```python
from build123d import *

# Parameters (mm, degrees)
SKETCH_1_R      = 98
SKETCH_1_R_2    = 47
EXTRUDE_1_DEPTH = 20
SKETCH_2_W      = 142.329371157
SKETCH_2_H      = 73.846071027
EXTRUDE_2_DEPTH = 15
FILLET_1_R      = 22


with BuildPart() as part:
    # 草图1 → 凸台-拉伸1 (new body)
    with BuildSketch(Plane.XY):
        with Locations((-11.887359686, -2.794806673)):
            Circle(SKETCH_1_R)
        with Locations((-11.887359686, -2.794806673)):
            Circle(SKETCH_1_R_2, mode=Mode.SUBTRACT)
    extrude(amount=EXTRUDE_1_DEPTH)

    # 草图2 → 凸台-拉伸2 (add)
    with BuildSketch(Plane.XY.offset(20)):
        with Locations((-173.83028852, -2.794806673)):
            Rectangle(SKETCH_2_W, SKETCH_2_H)
    extrude(amount=-EXTRUDE_2_DEPTH)

    # 圆角1
    fillet_1_edges = [part.edges().sort_by_distance(p)[0] for p in [
        (-102.665602941, 34.128228841, 12.5),
        (-102.665602941, -39.717842186, 12.5),
    ]]
    fillet(fillet_1_edges, radius=FILLET_1_R)


solid = part.part
```
Read the model definition and answer for the solid it produces. Units are mm, in the model's axes. A direction names the side the tool comes from. Give positions to 0.01 mm unless a question says otherwise; leave off trailing zeros. Loops run counter-clockwise (first coordinate to the right, second up) from the corner with the lowest first, then second, coordinate; pieces in that order, holes last.
Item 1: For faces 4 (the flat face through (-182, -39.718, 13)), 5 (the flat face through (-244.995, -3, 13)), 6 (the flat face through (-182, 34.128, 13)), determine the directions among +Z, -Z, +X, -X, +Y, -Y from which every point of the face is accessible in a straight line to the end or side of a thin tool.
Item 2: Each of these flat-tipped pins is pushed along its axis until it touches: pin 1 Ø3 at (y, z) = (69.5, 3) entering from -X; pin 2 Ø8 at (x, y) = (-198, 14.5) entering from -Z; pin 3 Ø3 at (x, z) = (-168.5, 4.5) entering from +Y. Where does it stop, or does it pass through?
Item 3: Find the intervals of material crossed by line 1 along Y through (x, z) = (-54, 8); line 2 along X through (y, z) = (-25.5, 1.75); line 3 along Y through (x, z) = (-0.5, 15.75), in increasing order.
Item 4: The part is cut by section A-A (x = 24). Write down the section's boundary in (y, z), and give its area (3 significant figures).
Item 5: The part is cut by section D-D (x = -199). Write down the section's boundary in (y, z), and give its area (3 significant figures).
Item 6: The mould has two halves that part along Y. Classify faces 1 (the flat face through (30, 20, 0)), 2 (the cylindrical face through (-18.006, 43.805, 9.86)), 3 (the cylindrical face through (-105.47, -42.64, 12.4)): released by +Y, released by -Y, zero draft, split by the parting line, or undercut.
Item 7: The part is cut by section B-B (y = 31). Write down the section's boundary in (x, z).
Item 8: The part is cut by section C-C (z = 14.25). Write down the section's boundary in (x, y).
Taken from the geometry:
1. face 4: +Z, -Z, -X, -Y
1. face 5: +Z, -Z, -X, +Y, -Y
1. face 6: +Z, -Z, -X, +Y
2. pin 1: stops at x = -79.65
2. pin 2: stops at z = 5
2. pin 3: stops at y = 34.13
3. line 1: y = -91.29 to -23.66, 18.07 to 85.7
3. line 2: x = -107.22 to -53.04, 29.26 to 83.45
3. line 3: y = -100.13 to -48.39, 42.8 to 94.54
4. outline: (-93.99, 0) - (-33.14, 0) - (-33.14, 20) - (-93.99, 20) - close; (27.55, 0) - (88.4, 0) - (88.4, 20) - (27.55, 20) - close
4. area: 2,430 mm2
5. outline: (-39.72, 5) - (34.13, 5) - (34.13, 20) - (-39.72, 20) - close
5. area: 1,110 mm2
6. face 1: zero draft
6. face 2: undercut
6. face 3: released by -Y
7. outline: (-244.99, 5) - (-103.88, 5) - (-103.88, 0) - (-44.55, 0) - (-44.55, 20) - (-244.99, 20) - close; (20.78, 0) - (80.1, 0) - (80.1, 20) - (20.78, 20) - close
8. outline: (-244.99, -39.72) - (-116.42, -39.72) arc R22 cw to (-97.26, -50.92) arc R98 ccw (long way) to (-97.26, 45.33) arc R22 cw to (-116.42, 34.13) - (-244.99, 34.13) - close; hole circle Ø94 at (-11.89, -2.79)
